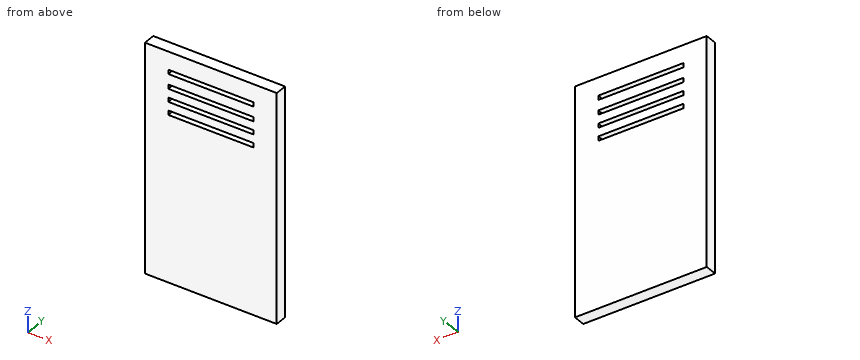
from build123d import *

# Parameters (mm, degrees)
F0_W     = 279.4
F0_H     = 482.6
F0_W_2   = 180.34
F0_H_2   = 9.333409
F0_H_3   = 9.09394
F0_H_4   = 9.093925
F1_DEPTH = 25.4
F2_DEPTH = 25.4


with BuildPart() as f1:
    # F0 (on Front) → F1 (new body)
    with BuildSketch(Plane.XZ):
        Rectangle(F0_W, F0_H)
        with Locations((-0.043589, 113.601674)):
            Rectangle(F0_W_2, F0_H_2, mode=Mode.SUBTRACT)
        with Locations((-0.043589, 140.737757)):
            Rectangle(F0_W_2, F0_H_3, mode=Mode.SUBTRACT)
        with Locations((-0.043589, 168.019548)):
            Rectangle(F0_W_2, F0_H_3, mode=Mode.SUBTRACT)
        with Locations((-0.043589, 198.938913)):
            Rectangle(F0_W_2, F0_H_4, mode=Mode.SUBTRACT)
    extrude(amount=F1_DEPTH)

    # F0 (on Front) → F2 (join)
    with BuildSketch(Plane.XZ):
        Rectangle(F0_W, F0_H)
        with Locations((-0.043589, 113.601674)):
            Rectangle(F0_W_2, F0_H_2, mode=Mode.SUBTRACT)
        with Locations((-0.043589, 140.737757)):
            Rectangle(F0_W_2, F0_H_3, mode=Mode.SUBTRACT)
        with Locations((-0.043589, 168.019548)):
            Rectangle(F0_W_2, F0_H_3, mode=Mode.SUBTRACT)
        with Locations((-0.043589, 198.938913)):
            Rectangle(F0_W_2, F0_H_4, mode=Mode.SUBTRACT)
    extrude(amount=F2_DEPTH)


solid = f1.part
Check sheet for the modelled part. Datum: model origin and axes. Units: mm. Give positions to 0.01 mm unless a question says otherwise; leave off trailing zeros. Loops run counter-clockwise (first coordinate to the right, second up) from the corner with the lowest first, then second, coordinate; pieces in that order, holes last. Notation, with made-up numbers: M 11.5,6 L 42.5,6 A28 cw 42.5,34 Z; hole C 31,88 d1. An arc over 180 degrees is marked long. Answer as a JSON object with one key per item and string values. Group by question number.
Q1. Cross-section at A-A on x = -40.5. Record the cut outline in (y, z).
Q2. Cross-section at B-B on y = -14.5. Record the cut outline in (x, z).
Q3. Material ranges on line 1 along Z through (x, y) = (12, -6.75); line 2 along X through (y, z) = (-5.75, 198.5), recorded low to high. Write a range as [from, to].
Q4. Go/stop test with a flat-tipped pin: P1, Ø1, axis at x = 65, z = -73.5, coming from the +Y side. Record where the tip stops, or that it passes through.
Evaluation:
{
 "1": {"outline": "M -25.4,-241.3 L 0,-241.3 L 0,108.93 L -25.4,108.93 Z; M -25.4,118.27 L 0,118.27 L 0,136.19 L -25.4,136.19 Z; M -25.4,145.28 L 0,145.28 L 0,163.47 L -25.4,163.47 Z; M -25.4,172.57 L 0,172.57 L 0,194.39 L -25.4,194.39 Z; M -25.4,203.49 L 0,203.49 L 0,241.3 L -25.4,241.3 Z"},
 "2": {"outline": "M -139.7,-241.3 L 139.7,-241.3 L 139.7,241.3 L -139.7,241.3 Z; hole M -90.21,108.93 L 90.13,108.93 L 90.13,118.27 L -90.21,118.27 Z; hole M -90.21,136.19 L 90.13,136.19 L 90.13,145.28 L -90.21,145.28 Z; hole M -90.21,163.47 L 90.13,163.47 L 90.13,172.57 L -90.21,172.57 Z; hole M -90.21,194.39 L 90.13,194.39 L 90.13,203.49 L -90.21,203.49 Z"},
 "3": {"line 1": "z = [-241.3, 108.93], [118.27, 136.19], [145.28, 163.47], [172.57, 194.39], [203.49, 241.3]", "line 2": "x = [-139.7, -90.21], [90.13, 139.7]"},
 "4": {"P1": "stops at y = 0"}
}
